Autodesk Inventor part; units mm, degrees
ref_plane "YZ Plane" through (0, 0, 0) normal (1, 0, 0) x (0, 1, 0)
ref_plane "XZ Plane" through (0, 0, 0) normal (0, 1, 0) x (-1, 0, 0)
ref_plane "XY Plane" through (0, 0, 0) normal (0, 0, 1) x (1, 0, 0)
sketch "Sketch1" plane through (0, 0, 0) normal (0, 0, 1) x (1, 0, 0)
  line L0 (-12.7, -12.7) -> (12.7, -12.7)
  line L1 (12.7, -12.7) -> (12.7, 12.7)
  line L2 (12.7, 12.7) -> (-12.7, 12.7)
  line L3 (-12.7, 12.7) -> (-12.7, -12.7)
  line L4 (-12.7, -12.7) -> (12.7, 12.7) construction
  line L5 (12.7, -12.7) -> (-12.7, 12.7) construction
  point P0 (0, 0)
  dimension "d0" = 25.4
  dimension "d1" = 25.4
extrude "Extrusion1" add sketch "Sketch1" along normal blind 609.6
fillet "Fillet1" radius 3.175 3 edges at (-12.7, -12.7, 304.8) (-12.7, 12.7, 304.8) (12.7, -12.7, 304.8)
fillet "Fillet2" radius 6.35 1 edges at (12.7, 12.7, 304.8)
properties part number "Lower Alignment"
Input: part model. Units: mm. Frame: model coordinates. Round coordinates to 2 decimals unless told otherwise and drop trailing zeros. Loops run counter-clockwise (first coordinate to the right, second up) from the corner with the lowest first, then second, coordinate; pieces in that order, holes last. Notation, with made-up numbers: M 74.25,-31.5 L 129.25,-31.5 A21 cw 129.25,5.5 Z; hole C -35.5,88.25 d11. An arc over 180 degrees is marked long. Answer in a Markdown table with one row per item. Add a question column.
1. Ray query, probe 1 along X at (y, z) = (-10, 554.5); probe 2 along X at (y, z) = (9.5, 369); probe 3 along Y at (x, z) = (9.25, 156). Return the intervals inside material, ascending.
2. Section A-A (z = 333). Output: boundary loops of the cut face in (x, y) (3 decimals).
3. Contact query for flat-ended pins moving along their axis: pin 1 (4 mm diameter, centred on y = 9.5, z = 188.5, fed in from +X) (3 decimals); pin 2 (1.5 mm diameter, centred on x = 10, z = 474.5, fed in from +Y). Output: stop coordinate, or through.
Values follow:
| question | item | result |
|---|---|---|
| 1 | probe 1 | -12.66 to 12.66 |
| 1 | probe 2 | -12.7 to 11.86 |
| 1 | probe 3 | -12.7 to 12 |
| 2 | outline | M -12.7,-9.525 A3.175 ccw -9.525,-12.7 L 9.525,-12.7 A3.175 ccw 12.7,-9.525 L 12.7,6.35 A6.35 ccw 6.35,12.7 L -9.525,12.7 A3.175 ccw -12.7,9.525 Z |
| 3 | pin 1 | x = 12.595 |
| 3 | pin 2 | y = 12 |
